from build123d import *

# Parameters (mm, degrees)
F0_W     = 19.05
F0_H     = 43.18
F1_DEPTH = 5.08
F2_R     = 1.202525
F3_DEPTH = 2.54
F4_R     = 1.488728
F5_DEPTH = 5.08
F6_R     = 1.27
F7_DEPTH = 25.4


with BuildPart() as f1:
    # F0 (on Front) → F1 (new body)
    with BuildSketch(Plane.XZ):
        Rectangle(F0_W, F0_H)
    extrude(amount=F1_DEPTH)

    # F2 (on face) → F3 (cut)
    with BuildSketch(Plane.YZ.offset(9.525)):
        with Locations((-2.590251, 11.43)):
            Circle(F2_R)
    extrude(amount=-F3_DEPTH, mode=Mode.SUBTRACT)

    # F4 (on face) → F5 (cut)
    with BuildSketch(Plane(origin=(-9.525, 0, 0), x_dir=(0, -1, 0), z_dir=(-1, 0, 0))):
        with Locations((2.54, 11.43)):
            Circle(F4_R)
    extrude(amount=-F5_DEPTH, mode=Mode.SUBTRACT)

    # F6 (on face) → F7 (cut)
    with BuildSketch(Plane.YZ.offset(9.525)):
        with Locations((-2.463937, 18.757666)):
            Circle(F6_R)
    extrude(amount=-F7_DEPTH, mode=Mode.SUBTRACT)


solid = f1.part
Build history of the part. All positions in model axes, mm. A direction names the side the tool comes from. Coordinates: 2 decimals unless noted, no trailing zeros. Order: outer loops, then holes, each group sorted by start corner. A loop starts at its lowest first (then second) coordinate and runs counter-clockwise, first axis right, second up. Notation, with made-up numbers: (26, 79) - (76, 79) arc R18 ccw to (76, 96) - close; hole circle Ø9 at (-1, 29.25). An arc over 180 degrees is marked (long way). Write each question's results on one line, items separated by ' | '. Start each with the question number.
Item 1: Band-saw the part on A-A on y = -2.54. Write the cut outline in (x, z) (3 decimals).
Item 2: Mould opens along Z. For faces 1 (the face through (-9.525, -3, 0)), 2 (the face through (0, -3, -21.59)), 3 (the face through (0.133, -2.629, 20.017)) say: released by +Z, released by -Z, zero draft, split by the parting line, or undercut.
Item 3: Tool access for faces 4 (the face through (0, 0, 0)), 5 (the face through (6.985, -3, 11)), 6 (the face through (-7.021, -2.217, 9.977)): list every direction of +Z, -Z, +X, -X, +Y, -Y with a clear straight run to the whole face (end or side of a thin tool).
Item 4: Band-saw the part on C-C on x = 3.25. Write the cut outline in (y, z), and give its area (3 significant figures).
Item 5: Band-saw the part on D-D on x = -6.25. Write the cut outline in (y, z).
Item 6: Band-saw the part on B-B on z = 11.43. Write the cut outline in (x, y) (3 decimals).
Item 7: Wall check: probe 1 along Z at (x, y) = (-7.5, -2.54); probe 2 along Z at (x, y) = (8.75, -2.6); probe 3 along Z at (x, y) = (0.5, -1.4). Give the ranges that are in metal, low to high. Write a range as [from, to].
Item 8: Flat gauge pin, fed straight in: pin 1 (0.9 mm diameter, centred on y = -2, z = 11.5, fed in from -X) (3 decimals). Where does the tip first touch, or does it go through?
Numbers:
1) outline: (-9.525, -21.59) - (9.525, -21.59) - (9.525, 10.229) - (6.985, 10.229) - (6.985, 12.631) - (9.525, 12.631) - (9.525, 17.49) - (-9.525, 17.49) - (-9.525, 12.919) - (-4.445, 12.919) - (-4.445, 9.941) - (-9.525, 9.941) - close; (-9.525, 20.025) - (9.525, 20.025) - (9.525, 21.59) - (-9.525, 21.59) - close
2) face 1: zero draft | face 2: released by -Z | face 3: undercut
3) face 4: +Z, -Z, +X, -X, +Y | face 5: +X | face 6: -X
4) outline: (-5.08, -21.59) - (0, -21.59) - (0, 21.59) - (-5.08, 21.59) - close; hole circle Ø2.54 at (-2.46, 18.76) | area: 214 mm^2
5) outline: (-5.08, -21.59) - (0, -21.59) - (0, 21.59) - (-5.08, 21.59) - close; hole circle Ø2.98 at (-2.54, 11.43); hole circle Ø2.54 at (-2.46, 18.76)
6) outline: (-9.525, -5.08) - (9.525, -5.08) - (9.525, -3.793) - (6.985, -3.793) - (6.985, -1.388) - (9.525, -1.388) - (9.525, 0) - (-9.525, 0) - (-9.525, -1.051) - (-4.445, -1.051) - (-4.445, -4.029) - (-9.525, -4.029) - close
7) probe 1: [-21.59, 9.94], [12.92, 17.49], [20.03, 21.59] | probe 2: [-21.59, 10.23], [12.63, 17.49], [20.02, 21.59] | probe 3: [-21.59, 18.06], [19.45, 21.59]
8) pin 1: x = -4.445
